```python
from build123d import *

# Parameters (mm, degrees)
F2_R = 1
F3_R = 5


with BuildPart() as f1:
    # F0 (on Front) → F1 (revolve)
    with BuildSketch(Plane.XZ):
        Polygon((0, -10), (0, 10), (-6, 10), (-2.5, 0), (-6, -10), align=None)
    revolve(axis=Axis((0, 0, 0), (0, 0, -1)))

    # F2
    f2_edges = [f1.edges().sort_by_distance(p)[0] for p in [
        (6, 0, 10),
        (6, 0, -10),
    ]]
    fillet(f2_edges, radius=F2_R)

    # F3
    f3_edges = [f1.edges().sort_by_distance(p)[0] for p in [
        (2.5, 0, 0),
    ]]
    fillet(f3_edges, radius=F3_R)


solid = f1.part
```
Model file for the job. Use its own axes, mm. Give positions to 0.01 mm unless a question says otherwise; leave off trailing zeros. Order: outer loops, then holes, each group sorted by start corner. A loop starts at its lowest first (then second) coordinate and runs counter-clockwise, first axis right, second up.
1) Pin check, flat tips, straight feed: pin 1 (1 mm diameter, centred on x = -1, z = 5.5, fed in from +Y); pin 2 (1.5 mm diameter, centred on y = 0.5, z = 1.5, fed in from +X); pin 3 (2 mm diameter, centred on x = 3, z = 2, fed in from +Y). Stop position of each tip, or through.
2) Saw through at B-B, the plane z = -6. Write the cut outline in (x, y), then the cut area to 3 significant figures.
3) Wall check: probe 1 along Y at (x, z) = (-1.5, -8.75); probe 2 along X at (y, z) = (-0.25, -2); probe 3 along Z at (x, y) = (2.5, 3.5). Give the ranges that are in metal, low to high.
4) Mould opens along Z. For faces 1 (the flat face through (0, 0, -10)), 2 (the flat face through (0, 0, 10)), 3 (the conical face through (-3.57, 1.12, 3.55)) say: +Z half, -Z half, draft (parallel to the pull), parting line (faces both ways), or undercut.
5) Saw through at A-A, the plane z = -4. Write the cut outline in (x, y).
Computed:
1. pin 1: stops at y = 4.52
1. pin 2: stops at x = 3.26
1. pin 3: stops at y = 2.61
2. outline: circle Ø9.2 at (0, 0)
2. area: 66.5 mm2
3. probe 1: y = -5.35 to 5.35
3. probe 2: x = -3.19 to 3.19
3. probe 3: z = -10 to -5.15, 5.15 to 10
4. face 1: -Z half
4. face 2: +Z half
4. face 3: undercut
5. outline: circle Ø7.8 at (0, 0)
